For this review, take the finished solid that the model builds, in its own axes (mm). A direction names the side the tool comes from. Round coordinates to 2 decimals unless told otherwise and drop trailing zeros. Loops run counter-clockwise (first coordinate to the right, second up) from the corner with the lowest first, then second, coordinate; pieces in that order, holes last.
1) Take a section at A-A (z = 3). State the section outline as (x, y) points.
2) Insertion check: pin 1 (10 mm diameter, centred on x = 78, y = 25, fed in from -Z); pin 2 (1.5 mm diameter, centred on x = 78, z = 26, fed in from -Y); pin 3 (19 mm diameter, centred on x = 57.93, y = 32.65, fed in from +Z). Each pin has a flat end and moves straight along its axis. Give the tip position at first contact, or say it passes through.
3) Take a section at C-C (x = 86.5). State the section outline as (y, z) points.
4) Tool access review of faces 1 (the cylindrical face through (6.54, 34.64, 27.79)), 2 (the flat face through (53, 1, 0)): name each direction out of +Z, -Z, +X, -X, +Y, -Y from which nothing blocks a thin tool from reaching the whole face with its end or side.
5) Take a section at D-D (x = 49.5). State the section outline as (y, z) points.
6) Wall thickness on L1, parallel to Y at x = 78.5, z = 2; L2, parallel to X at y = 36.5, z = 13; L3, parallel to Z at x = 58.5, y = 21: over which ranges is each line inside the solid? List them lowest first.
7) Take a section at B-B (y = 27). State the section outline as (x, z) points, then the cut area to 3 significant figures.
8) Mouldability with a two-part tool opening along X and no side actions: class faces 3 (the cylindrical face through (58.736, 4.721, 29.565)), 4 (the flat face through (113.31, 34, 9)), 5 (the flat face through (0, 34, 9)) as pulls with the +X half, pulls with the -X half, needs draft (parallel to the pull), parting line crosses it, or undercut.
```python
from build123d import *

# Parameters (mm, degrees)
F0_W     = 115.850285
F0_H     = 68.390653
F1_DEPTH = 34.544
F2_R     = 16.556677
F3_T     = -2.54
F4_R     = 10.511937
F5_DEPTH = 25.4


with BuildPart() as f1:
    # F0 (on Top) → F1 (new body)
    with BuildSketch(Plane.XY):
        with Locations((57.925142, 34.195327)):
            Rectangle(F0_W, F0_H)
    extrude(amount=F1_DEPTH)

    # F2
    f2_edges = [f1.edges().sort_by_distance(p)[0] for p in [
        (0, 34.195326, 34.544),
        (57.925142, 0, 34.544),
        (115.850285, 34.195326, 34.544),
        (57.925142, 68.390653, 34.544),
    ]]
    fillet(f2_edges, radius=F2_R)

    # F3
    f3_openings = [f1.faces().sort_by_distance(p)[0] for p in [
        (57.925142, 34.195326, 0),
    ]]
    offset(amount=F3_T, openings=f3_openings)

    # F4 (on face) → F5 (cut)
    with BuildSketch(Plane.XY.offset(34.544)):
        with Locations((57.925142, 32.649688)):
            Circle(F4_R)
    extrude(amount=-F5_DEPTH, mode=Mode.SUBTRACT)


solid = f1.part
```
Response:
1. outline: (0, 0) - (115.85, 0) - (115.85, 68.39) - (0, 68.39) - close; hole (2.54, 2.54) - (113.31, 2.54) - (113.31, 65.85) - (2.54, 65.85) - close
2. pin 1: stops at z = 32
2. pin 2: stops at y = 1.68
2. pin 3: passes through
3. outline: (0, 0) - (2.54, 0) - (2.54, 17.99) arc R14.02 cw to (16.56, 32) - (51.83, 32) arc R14.02 cw to (65.85, 17.99) - (65.85, 0) - (68.39, 0) - (68.39, 17.99) arc R16.56 ccw to (51.83, 34.54) - (16.56, 34.54) arc R16.56 ccw to (0, 17.99) - close
4. face 1: -Z
4. face 2: -Z, +X, -X, +Y, -Y
5. outline: (0, 0) - (2.54, 0) - (2.54, 17.99) arc R14.02 cw to (16.56, 32) - (26.36, 32) - (26.36, 34.54) - (16.56, 34.54) arc R16.56 ccw to (0, 17.99) - close; (38.94, 32) - (51.83, 32) arc R14.02 cw to (65.85, 17.99) - (65.85, 0) - (68.39, 0) - (68.39, 17.99) arc R16.56 ccw to (51.83, 34.54) - (38.94, 34.54) - close
6. L1: y = 0 to 2.54, 65.85 to 68.39
6. L2: x = 0 to 2.54, 113.31 to 115.85
6. L3: z = 32 to 34.54
7. outline: (0, 0) - (2.54, 0) - (2.54, 17.99) arc R14.02 cw to (16.56, 32) - (49.06, 32) - (49.06, 34.54) - (16.56, 34.54) arc R16.56 ccw to (0, 17.99) - close; (66.79, 32) - (99.29, 32) arc R14.02 cw to (113.31, 17.99) - (113.31, 0) - (115.85, 0) - (115.85, 17.99) arc R16.56 ccw to (99.29, 34.54) - (66.79, 34.54) - close
7. area: 378 mm2
8. face 3: needs draft
8. face 4: undercut
8. face 5: pulls with the -X half
